Read the model definition and answer for the solid it produces. Units are mm, in the model's axes. A direction names the side the tool comes from. Give positions to 0.01 mm unless a question says otherwise; leave off trailing zeros. Loops run counter-clockwise (first coordinate to the right, second up) from the corner with the lowest first, then second, coordinate; pieces in that order, holes last. Notation, with made-up numbers: M 22.5,-5 L 46.5,-5 A8 cw 46.5,0 Z; hole C 71,62.25 d3. An arc over 180 degrees is marked long. Return JSON: item names as keys, results as strings. Group by question number.
```python
from build123d import *

# Parameters (mm, degrees)
BOSS_EXTRUDE1_DEPTH = 2.5
SKETCH3_W           = 50
SKETCH3_H           = 1.25
CUT_EXTRUDE2_DEPTH  = 1.25
CHAMFER2_SIZE       = 1.25


with BuildPart() as part:
    # Sketch1 → Boss-Extrude1 (new body)
    with BuildSketch(Plane(origin=(0, 0, 0), x_dir=(1, 0, 0), z_dir=(0, 1, 0))):
        with BuildLine():
            Line((0, 0), (-8.75, 0))
            ThreePointArc((-8.75, 0), (-6.187184335, 6.187184335), (0, 8.75))
            Line((0, 8.75), (50, 8.75))
            ThreePointArc((50, 8.75), (56.187184335, 6.187184335), (58.75, 0))
            Line((58.75, 0), (50, 0))
            Line((50, 0), (0, 0))
        make_face()
    extrude(amount=BOSS_EXTRUDE1_DEPTH)

    # Sketch3 → Cut-Extrude2 (cut)
    with BuildSketch(Plane.XZ):
        with BuildLine():
            Line((58.75, 0), (57.5, 0))
            ThreePointArc((57.5, 0), (55.303300859, -5.303300859), (50, -7.5))
            Line((50, -7.5), (50, -8.75))
            ThreePointArc((50, -8.75), (56.187184335, -6.187184335), (58.75, 0))
        make_face()
        with Locations((25, -8.125)):
            Rectangle(SKETCH3_W, SKETCH3_H)
        with BuildLine():
            Line((-7.5, 0), (-8.75, 0))
            ThreePointArc((-8.75, 0), (-6.187184335, -6.187184335), (0, -8.75))
            Line((0, -8.75), (0, -7.5))
            ThreePointArc((0, -7.5), (-5.303300859, -5.303300859), (-7.5, 0))
        make_face()
    extrude(amount=-CUT_EXTRUDE2_DEPTH, mode=Mode.SUBTRACT)

    # Chamfer2
    chamfer2_edges = [part.edges().sort_by_distance(p)[0] for p in [
        (56.187184335, 1.25, -6.187184335),
        (25, 1.25, -8.75),
        (-6.187184335, 1.25, -6.187184335),
    ]]
    chamfer(chamfer2_edges, length=CHAMFER2_SIZE - 0.0001)  # a hair under: the kernel refuses the full size


solid = part.part
```
1. Straight lines are drawn through the part: line 1 along Z through (x, y) = (9.5, 1.1); line 2 along Z through (x, y) = (1, 2.3); line 3 along X through (y, z) = (1.85, -5.25). For each, find the intervals that lie inside material, in ascending order.
2. For faces 1 (the flat face through (25, 1, -7.5)), 2 (the cylindrical face through (-5.245, 0.616, -5.361)), 3 (the cylindrical face through (55.361, 0.616, -5.245)), determine the directions among +Z, -Z, +X, -X, +Y, -Y from which every point of the face is accessible in a straight line to the end or side of a thin tool.
3. A flat-ended cylindrical pin translates along its axis: P1, Ø4, axis at x = 31, z = -6, coming from the -Y side. Find the tip coordinate at first contact, or state that the pin passes through.
4. Find section B-B (y = 0.7). Write down the section's boundary in (x, z), and give its area (3 significant figures).
Result:
{
 "1": {"line 1": "z = -7.5 to 0", "line 2": "z = -8.55 to 0", "line 3": "x = -6.17 to 56.17"},
 "2": {"face 1": "-Z, +X, -X, -Y", "face 2": "-Z, -X, -Y", "face 3": "-Z, +X, -Y"},
 "3": {"P1": "stops at y = 0"},
 "4": {"outline": "M -7.5,0 A7.5 ccw 0,-7.5 L 50,-7.5 A7.5 ccw 57.5,0 Z", "area": "463 mm2"}
}
